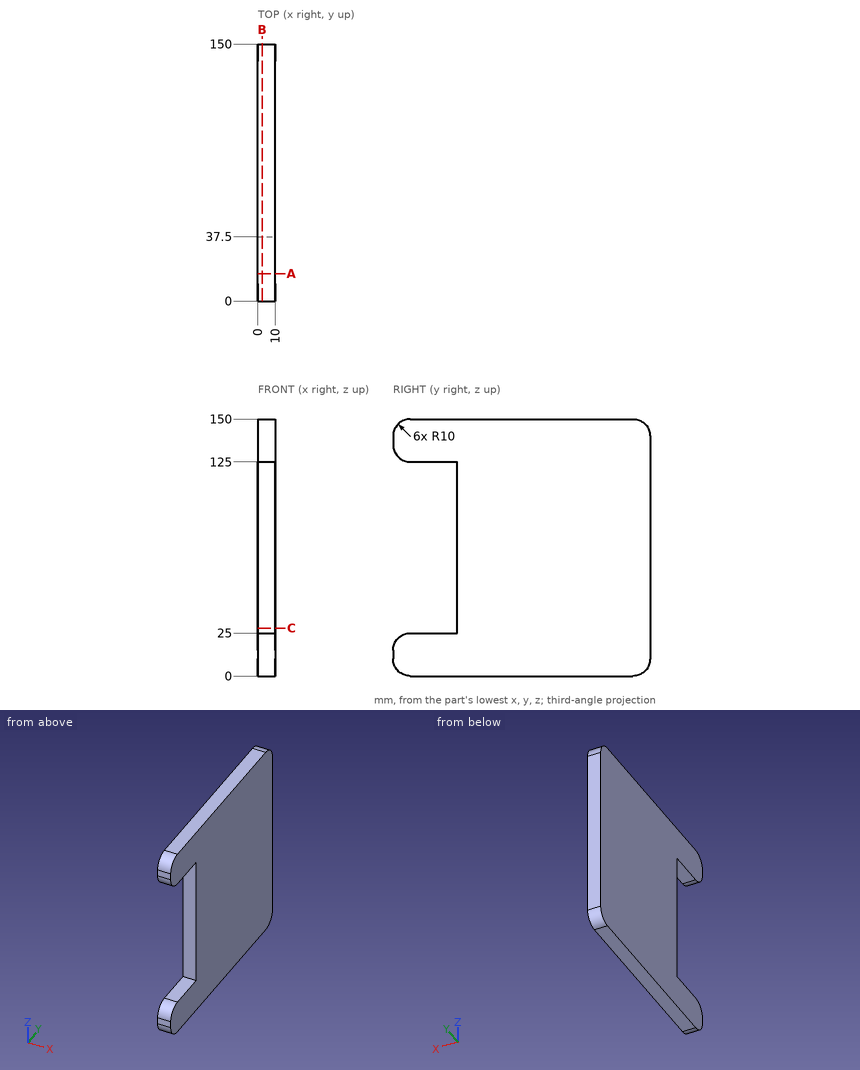
Verification items for this drawing (mm, ordinates from the low corner). Give positions to 0.01 mm unless a question says otherwise; leave off trailing zeros. Write each loop counter-clockwise with the first axis right and the second up, starting at its lowest first coordinate (ties: lowest second). Pieces come first, ordered by that corner, then holes. Notation, with made-up numbers: (-39.5, 14.5) -> (-12.5, 14.5) arc R11 cw to (-12.5, 19.5) -> close; hole circle Ø3 at (-26, 27). An arc over 180 degrees is marked (long way). Use CSV: the item, a comma, the result in double quotes.
(1) Sectioned sample at A-A (y = 16). Record the cut outline in (x, z), plus the area to 3 significant figures.
Derived:
outline,"(0, 0) -> (10, 0) -> (10, 25) -> (0, 25) -> close; (0, 125) -> (10, 125) -> (10, 150) -> (0, 150) -> close"
area,"500 mm^2"
(2) Sectioned sample at C-C (z = 28). Record the cut outline in (x, y), plus the area to 4 significant figures.
Derived:
outline,"(0, 37.5) -> (10, 37.5) -> (10, 150) -> (0, 150) -> close"
area,"1,125 mm^2"
(3) Material ranges on L1, parallel to Z at x = 9.5, y = 27; L2, parallel to Y at x = 4.5, z = 31; L3, parallel to Y at x = 4.5, z = 132, recorded low to high.
Derived:
L1,"z = 0 to 25, 125 to 150"
L2,"y = 37.5 to 150"
L3,"y = 0.46 to 150"
(4) Sectioned sample at B-B (x = 2.5). Record the cut outline in (y, z), plus the area to 3 significant figures.
Derived:
outline,"(0, 10) arc R10 ccw to (10, 0) -> (140, 0) arc R10 ccw to (150, 10) -> (150, 140) arc R10 ccw to (140, 150) -> (10, 150) arc R10 ccw to (0, 140) -> (0, 135) arc R10 ccw to (10, 125) -> (37.5, 125) -> (37.5, 25) -> (10, 25) arc R10 ccw to (0, 15) -> close"
area,"18,600 mm^2"
(5) Go/stop test with a flat-tipped pin: pin 1 (3 mm diameter, centred on x = 5.5, z = 120.5, fed in from -Y). Record where the tip stops, or that it passes through.
Derived:
pin 1,"stops at y = 37.5"
